Verification items for this drawing (mm, ordinates from the low corner). Round coordinates to 2 decimals unless told otherwise and drop trailing zeros. Write each loop counter-clockwise with the first axis right and the second up, starting at its lowest first coordinate (ties: lowest second). Pieces come first, ordered by that corner, then holes.
Item 1: Draft check along X on the marked faces 1, 2, 3 and 4. Enter one of: pulls with the +X half, pulls with the -X half, needs draft (parallel to the pull), parting line crosses it, or undercut.
Item 2: Depth check by flat-ended pin: P1, Ø2, axis at y = 15, z = 4, coming from the -X side; P2, Ø2, axis at x = 7.6, z = 3.675, coming from the -Y side; P3, Ø5, axis at y = 16, z = 12, coming from the +X side; P4, Ø6, axis at x = 7.5, y = 8.5, coming from the -Z side. Enter the tip coordinate at first touch or a pass-through.
Item 3: Cross-section at B-B (z = 7.6). Enter the section's corners in (x, y).
Item 4: Scan lines: probe 1 along Z at (x, y) = (7.6, 1.65) (3 decimals); probe 2 along Z at (x, y) = (7.6, 16.25); probe 3 along X at (y, z) = (10.5, 8.5). Record each from-to range of solid material in increasing order.
Item 5: Cross-section at C-C (y = 20). Enter the section's corners in (x, z).
Item 6: Cross-section at D-D (z = 11.75). Enter the section's corners in (x, y), then the cut area to 3 significant figures.
Item 7: Cross-section at A-A (x = 7.6). Enter the section's corners in (y, z) (3 decimals).
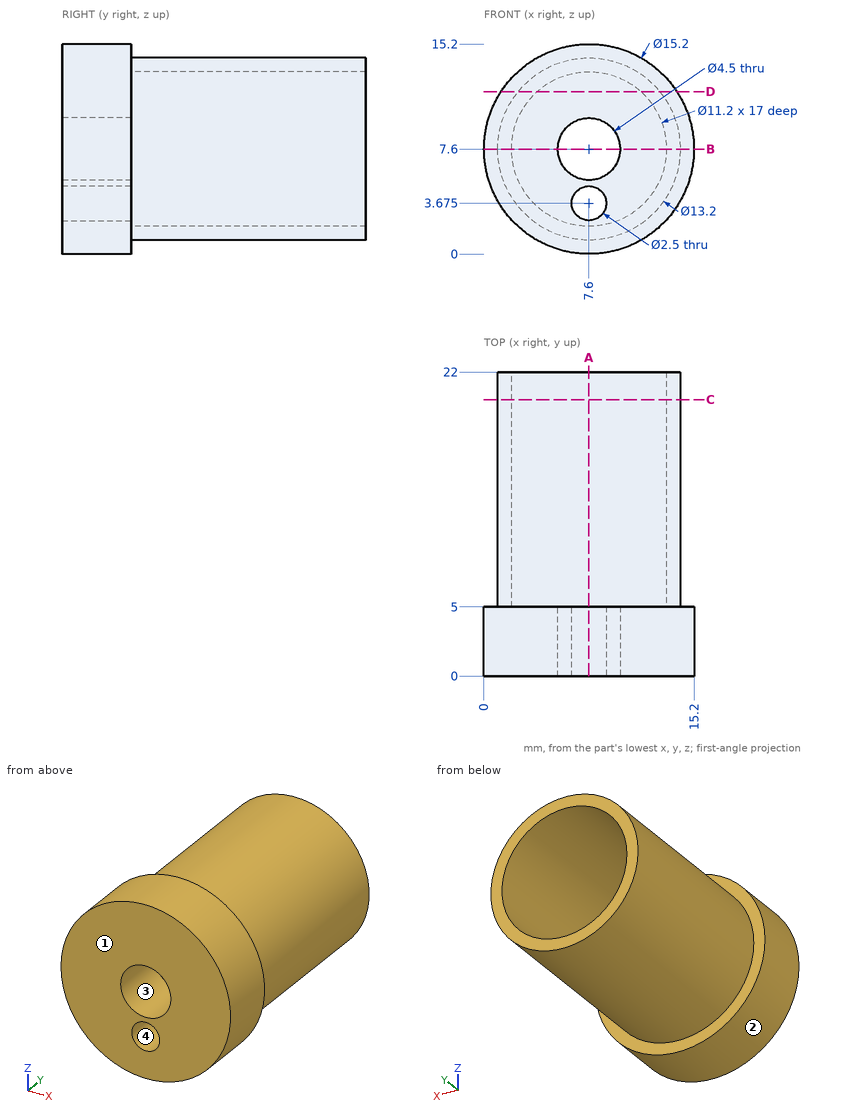
Resolved:
1. face 1: needs draft
1. face 2: parting line crosses it
1. face 3: undercut
1. face 4: undercut
2. P1: stops at x = 1.53
2. P2: passes through
2. P3: stops at x = 13.92
2. P4: stops at z = 1
3. outline: (0, 0) - (5.35, 0) - (5.35, 5) - (2, 5) - (2, 22) - (1, 22) - (1, 5) - (0, 5) - close; (9.85, 0) - (15.2, 0) - (15.2, 5) - (14.2, 5) - (14.2, 22) - (13.2, 22) - (13.2, 5) - (9.85, 5) - close
4. probe 1: z = 0 to 2.425, 4.925 to 5.35, 9.85 to 15.2
4. probe 2: z = 1 to 2, 13.2 to 14.2
4. probe 3: x = 1.06 to 2.07, 13.13 to 14.14
5. outline: circle Ø13.2 at (7.6, 7.6); hole circle Ø11.2 at (7.6, 7.6)
6. outline: (1.23, 0) - (13.97, 0) - (13.97, 5) - (12.73, 5) - (12.73, 22) - (11.36, 22) - (11.36, 5) - (3.84, 5) - (3.84, 22) - (2.47, 22) - (2.47, 5) - (1.23, 5) - close
6. area: 110 mm2
7. outline: (0, 0) - (5, 0) - (5, 1) - (22, 1) - (22, 2) - (5, 2) - (5, 2.425) - (0, 2.425) - close; (0, 4.925) - (5, 4.925) - (5, 5.35) - (0, 5.35) - close; (0, 9.85) - (5, 9.85) - (5, 13.2) - (22, 13.2) - (22, 14.2) - (5, 14.2) - (5, 15.2) - (0, 15.2) - close
